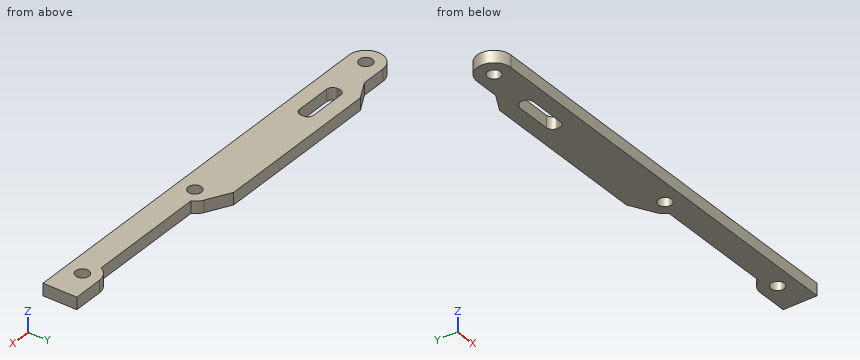
```python
from build123d import *

# Parameters (mm, degrees)
SKETCH1_R           = 1.65
BOSS_EXTRUDE1_DEPTH = 3
FILLET1_R           = 1.5


with BuildPart() as part:
    # Sketch1 → Boss-Extrude1 (new body)
    with BuildSketch(Plane.XY):
        with BuildLine():
            Line((-57, -4.2), (45, -4.2))
            Line((45, -4.2), (45, 4.2))
            Line((45, 4.2), (37.5, 4.2))
            ThreePointArc((37.5, 4.2), (35.255005568, 3.54964787), (33.705266808, 1.8))
            Line((33.705266808, 1.8), (3.794733192, 1.8))
            ThreePointArc((3.794733192, 1.8), (3.042029577, 2.89586879), (1.984520956, 3.701577579))
            Line((1.984520956, 3.701577579), (-3.794733192, 6.8))
            Line((-3.794733192, 6.8), (-46, 6.8))
            Line((-46, 6.8), (-50.849584319, 4.2))
            Line((-50.849584319, 4.2), (-57, 4.2))
            ThreePointArc((-57, 4.2), (-61.2, 0), (-57, -4.2))
        make_face()
        Circle(SKETCH1_R, mode=Mode.SUBTRACT)
        with Locations((-57, 0)):
            Circle(SKETCH1_R, mode=Mode.SUBTRACT)
        with Locations((37.5, 0)):
            Circle(SKETCH1_R, mode=Mode.SUBTRACT)
        Polygon((-46, -0.45), (-34, -0.45), (-34, 1.8), (-34, 3.05), (-46, 3.05), (-46, 1.8), align=None, mode=Mode.SUBTRACT)
    extrude(amount=BOSS_EXTRUDE1_DEPTH)

    # Fillet1
    fillet1_edges = [part.edges().sort_by_distance(p)[0] for p in [
        (-34, -0.45, 1.5),
        (-34, 3.05, 1.5),
        (-46, 3.05, 1.5),
        (-46, -0.45, 1.5),
    ]]
    fillet(fillet1_edges, radius=FILLET1_R)


solid = part.part
```
Verification items for the finished model (mm, model axes). Give positions to 0.01 mm unless a question says otherwise; leave off trailing zeros. Order: outer loops, then holes, each group sorted by start corner. A loop starts at its lowest first (then second) coordinate and runs counter-clockwise, first axis right, second up. Notation, with made-up numbers: (-37, 43.5) -> (-5, 43.5) arc R29 ccw to (-5, 77.5) -> close; hole circle Ø4 at (4.25, -6). An arc over 180 degrees is marked (long way). One line per item, written item: value.
(1) Sectioned sample at C-C on x = 0. Record the cut outline in (y, z).
Final values:
outline: (-4.2, 0) -> (-1.65, 0) -> (-1.65, 3) -> (-4.2, 3) -> close; (1.65, 0) -> (4.77, 0) -> (4.77, 3) -> (1.65, 3) -> close
(2) Sectioned sample at B-B on z = 0.5. Record the cut outline in (x, y), then the cut area to 3 significant figures.
Final values:
outline: (-57, -4.2) -> (45, -4.2) -> (45, 4.2) -> (37.5, 4.2) arc R4.2 ccw to (33.71, 1.8) -> (3.79, 1.8) arc R4.2 ccw to (1.98, 3.7) -> (-3.79, 6.8) -> (-46, 6.8) -> (-50.85, 4.2) -> (-57, 4.2) arc R4.2 ccw to start; hole circle Ø3.3 at (-57, 0); hole (-46, 1.05) arc R1.5 ccw to (-44.5, -0.45) -> (-35.5, -0.45) arc R1.5 ccw to (-34, 1.05) -> (-34, 1.55) arc R1.5 ccw to (-35.5, 3.05) -> (-44.5, 3.05) arc R1.5 ccw to (-46, 1.55) -> close; hole circle Ø3.3 at (0, 0); hole circle Ø3.3 at (37.5, 0)
area: 864 mm^2
(3) Gauge pin test, flat ends, axial feed: pin 1 (5 mm diameter, centred on x = 33, y = 4.5, fed in from -Z); pin 2 (1 mm diameter, centred on x = 6, z = 2, fed in from +Y); pin 3 (3 mm diameter, centred on x = 37.5, y = 0, fed in from -Z); pin 4 (1.5 mm diameter, centred on y = 3, z = 2, fed in from -X). Record the tip position at first contact, or that the pin passes through.
Final values:
pin 1: z = 0
pin 2: y = 1.8
pin 3: through
pin 4: x = -60.55
(4) Sectioned sample at A-A on x = -43. Record the cut outline in (y, z).
Final values:
outline: (-4.2, 0) -> (-0.45, 0) -> (-0.45, 3) -> (-4.2, 3) -> close; (3.05, 0) -> (6.8, 0) -> (6.8, 3) -> (3.05, 3) -> close
(5) Scan lines: line 1 along Y through (x, z) = (37.5, 0.8); line 2 along X through (y, z) = (-1.5, 1.1); line 3 along X through (y, z) = (1, 2.15). Record each from-to range of solid material in increasing order. Write a range as [from, to].
Final values:
line 1: [-4.2, -1.65], [1.65, 4.2]
line 2: [-60.92, -57.69], [-56.31, -0.69], [0.69, 36.81], [38.19, 45]
line 3: [-61.08, -58.31], [-55.69, -46], [-34, -1.31], [1.31, 36.19], [38.81, 45]
(6) Sectioned sample at D-D on y = 5.5. Record the cut outline in (x, z), then the cut area to 3 significant figures.
Final values:
outline: (-48.42, 0) -> (-1.37, 0) -> (-1.37, 3) -> (-48.42, 3) -> close
area: 141 mm^2
